Input: part model. Units: mm. Frame: model coordinates. Coordinates: 2 decimals unless noted, no trailing zeros. Loops run counter-clockwise (first coordinate to the right, second up) from the corner with the lowest first, then second, coordinate; pieces in that order, holes last.
(1) Contact query for flat-ended pins moving along their axis: P1, Ø2, axis at x = -26.5, z = 5, coming from the -Y side; P2, Ø1.9, axis at y = 3, z = 3, coming from the +X side. Output: stop coordinate, or through.
(2) Section B-B, the plane x = 0. Return loops of the section in (y, z).
(3) Section A-A, the plane y = 0. Return loops of the section in (x, z), then the cut area to 3 significant figures.
(4) Section D-D, the plane x = 42. Return loops of the section in (y, z).
(5) Line query: L1, parallel to Y at x = 0, z = 2.5; L2, parallel to Y at x = -0.5, z = 4; L3, parallel to Y at x = 18, z = 5.5. Output: solid intervals per line, ascending.
(6) Mould query, pull axis Y, two halves, no side actions, for faces 1 (the face through (11, -11, 0)), 2 (the face through (20.24, 35.24, 3.22)). Classes: released by +Y, released by -Y, zero draft, split by the parting line, or undercut.
(7) Section C-C, the plane x = -35.5. Return loops of the section in (y, z).
```python
from build123d import *

# Parameters (mm, degrees)
F0_R            = 50.8
F0_R_2          = 14.4272
F1_DEPTH        = 6.35
F2_W            = 12.7
F2_H            = 6.35
F3_DEPTH        = 6.351
F3_COPIES_COUNT = 12
F4_R            = 2.4892
F5_DEPTH        = 6.351
F5_COPIES_COUNT = 6


# Not quite as in the source:
# - a pattern or mirror of a feature is missing from the dataset's text; its kind, count and spacing are read off the source's solid


with BuildPart() as f1:
    # F0 (on Top) → F1 (new body)
    with BuildSketch(Plane.XY):
        Circle(F0_R)
        Circle(F0_R_2, mode=Mode.SUBTRACT)
    extrude(amount=F1_DEPTH)

    # F2 (on face) → F3 (cut, through all)
    with BuildSketch(Plane.XY.offset(6.35)):
        with Locations((0, 43.815)):
            Rectangle(F2_W, F2_H)
    f3 = extrude(amount=-F3_DEPTH, mode=Mode.SUBTRACT)

    # F3_copies: F3 ×12 about axis
    f3_copies_axis = Axis((0, 0, 0), (0, 0, 1))
    for i in range(1, F3_COPIES_COUNT):
        add(f3.rotate(f3_copies_axis, i * 360 / F3_COPIES_COUNT), mode=Mode.SUBTRACT)

    # F4 (on face) → F5 (cut, through all)
    with BuildSketch(Plane.XY.offset(6.35)):
        with Locations((0, 23.8125)):
            Circle(F4_R)
    f5 = extrude(amount=-F5_DEPTH, mode=Mode.SUBTRACT)

    # F5_copies: F5 ×6 about axis
    f5_copies_axis = Axis((0, 0, 0), (0, 0, 1))
    for i in range(1, F5_COPIES_COUNT):
        add(f5.rotate(f5_copies_axis, i * 360 / F5_COPIES_COUNT), mode=Mode.SUBTRACT)


solid = f1.part
```
Report:
1. P1: stops at y = -43.94
1. P2: stops at x = 50.76
2. outline: (-50.8, 0) - (-46.99, 0) - (-46.99, 6.35) - (-50.8, 6.35) - close; (-40.64, 0) - (-26.3, 0) - (-26.3, 6.35) - (-40.64, 6.35) - close; (-21.32, 0) - (-14.43, 0) - (-14.43, 6.35) - (-21.32, 6.35) - close; (14.43, 0) - (21.32, 0) - (21.32, 6.35) - (14.43, 6.35) - close; (26.3, 0) - (40.64, 0) - (40.64, 6.35) - (26.3, 6.35) - close; (46.99, 0) - (50.8, 0) - (50.8, 6.35) - (46.99, 6.35) - close
3. outline: (-50.8, 0) - (-46.99, 0) - (-46.99, 6.35) - (-50.8, 6.35) - close; (-40.64, 0) - (-14.43, 0) - (-14.43, 6.35) - (-40.64, 6.35) - close; (14.43, 0) - (40.64, 0) - (40.64, 6.35) - (14.43, 6.35) - close; (46.99, 0) - (50.8, 0) - (50.8, 6.35) - (46.99, 6.35) - close
3. area: 381 mm2
4. outline: (-28.58, 0) - (-21.23, 0) - (-21.23, 6.35) - (-28.58, 6.35) - close; (-16.92, 0) - (-6.35, 0) - (-6.35, 6.35) - (-16.92, 6.35) - close; (6.35, 0) - (16.92, 0) - (16.92, 6.35) - (6.35, 6.35) - close; (21.23, 0) - (28.58, 0) - (28.58, 6.35) - (21.23, 6.35) - close
5. L1: y = -50.8 to -46.99, -40.64 to -26.3, -21.32 to -14.43, 14.43 to 21.32, 26.3 to 40.64, 46.99 to 50.8
5. L2: y = -50.8 to -46.99, -40.64 to -26.25, -21.37 to -14.42, 14.42 to 21.37, 26.25 to 40.64, 46.99 to 50.8
5. L3: y = -47.5 to -43.87, -36.53 to 36.53, 43.87 to 47.5
6. face 1: zero draft
6. face 2: undercut
7. outline: (-36.34, 0) - (-27.83, 0) - (-27.83, 6.35) - (-36.34, 6.35) - close; (-19.79, 0) - (19.79, 0) - (19.79, 6.35) - (-19.79, 6.35) - close; (27.83, 0) - (36.34, 0) - (36.34, 6.35) - (27.83, 6.35) - close
